Geometry check sheet. Reference: drawing and pictorial views, mm from the part's lowest x, y, z. Round coordinates to 2 decimals unless told otherwise and drop trailing zeros. Order: outer loops, then holes, each group sorted by start corner. A loop starts at its lowest first (then second) coordinate and runs counter-clockwise, first axis right, second up. Notation, with made-up numbers: (48.5, 70) -> (92.5, 70) arc R22 cw to (92.5, 76) -> close; hole circle Ø2 at (-3, 22.25). An arc over 180 degrees is marked (long way). Put each result on its own line as item: value.
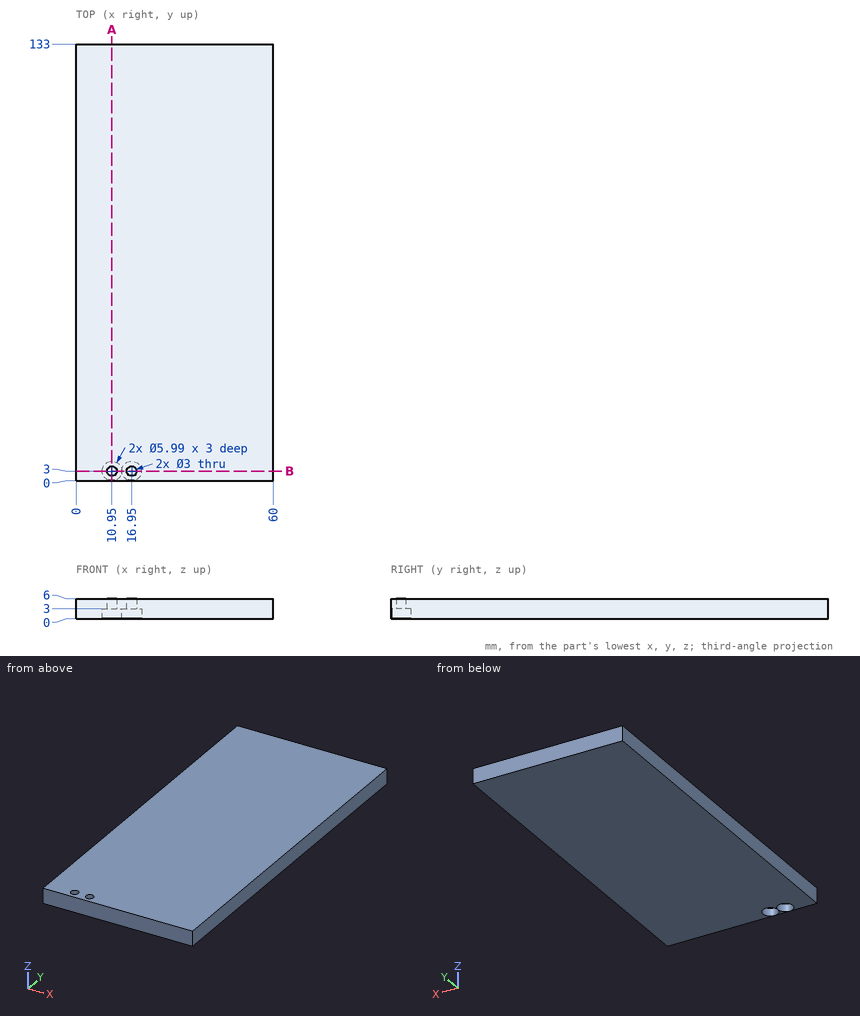
Item 1: Material ranges on line 1 along Y through (x, z) = (16.95, 5.1), recorded low to high.
Geometry check:
line 1: 0 to 1.5, 4.5 to 133
Item 2: Sectioned sample at A-A, the plane x = 10.95. Record the boundary of the cut face in (y, z) (3 decimals), then the cut area to 3 significant figures.
Geometry check:
outline: (0, 0) -> (0.005, 0) -> (0.005, 3) -> (1.5, 3) -> (1.5, 6) -> (0, 6) -> close; (4.5, 3) -> (5.995, 3) -> (5.995, 0) -> (133, 0) -> (133, 6) -> (4.5, 6) -> close
area: 771 mm2
Item 3: Depth check by flat-ended pin: pin 1 Ø2.5 at (x, y) = (10.95, 3) entering from +Z; pin 2 Ø3 at (x, y) = (17, 4) entering from -Z. Enter the tip coordinate at first touch or a pass-through.
Geometry check:
pin 1: through
pin 2: z = 3
Item 4: Sectioned sample at B-B, the plane y = 3. Record the boundary of the cut face in (x, z) (3 decimals), then the cut area to 3 significant figures.
Geometry check:
outline: (0, 0) -> (7.955, 0) -> (7.955, 3) -> (9.45, 3) -> (9.45, 6) -> (0, 6) -> close; (12.45, 3) -> (13.945, 3) -> (13.945, 0) -> (13.955, 0) -> (13.955, 3) -> (15.45, 3) -> (15.45, 6) -> (12.45, 6) -> close; (18.45, 3) -> (19.945, 3) -> (19.945, 0) -> (60, 0) -> (60, 6) -> (18.45, 6) -> close
area: 306 mm2
